The drawing under review shows one solid part. Ordinate dimensions are in mm from its lowest x, y, z. Coordinates: 2 decimals unless noted, no trailing zeros. Write each loop counter-clockwise with the first axis right and the second up, starting at its lowest first coordinate (ties: lowest second). Pieces come first, ordered by that corner, then holes.
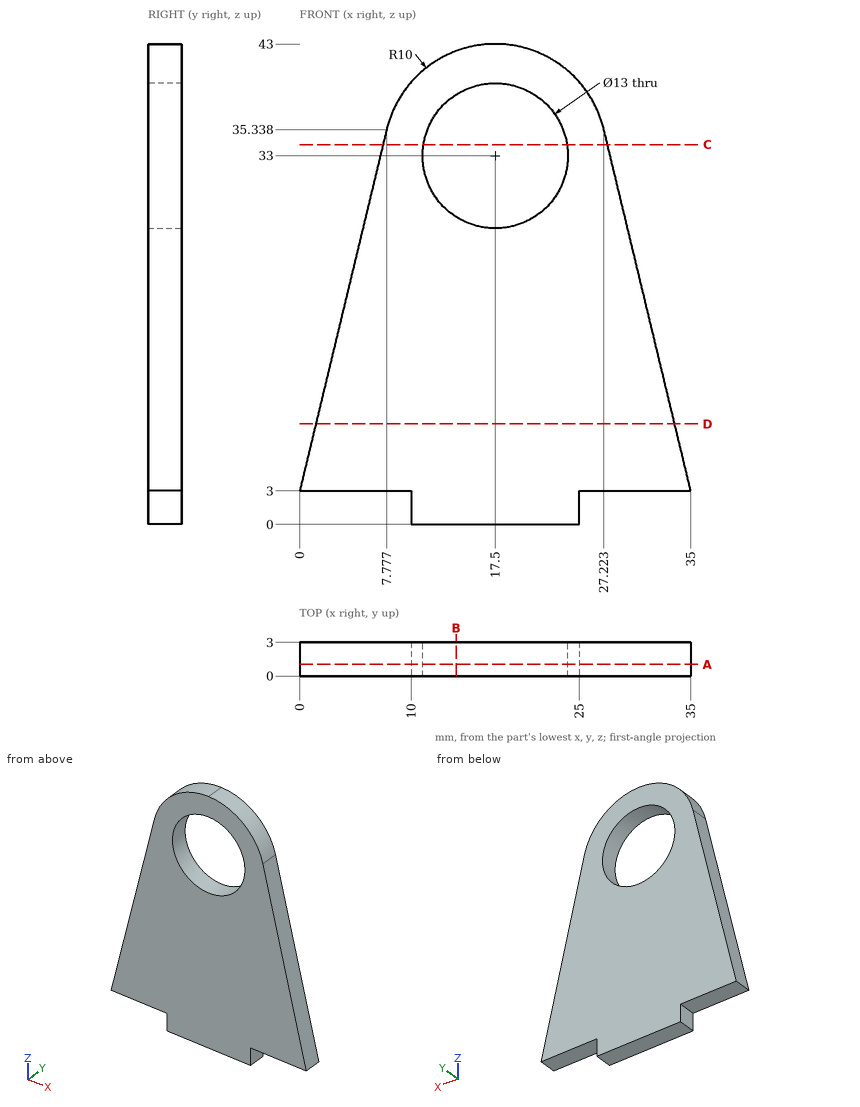
Q1. Add section A-A (y = 1.05). State the section outline as (x, z) points, then the cut area to 3 significant figures.
Ans:
outline: (0, 3) - (10, 3) - (10, 0) - (25, 0) - (25, 3) - (35, 3) - (27.22, 35.34) arc R10 ccw to (17.5, 43) arc R10 ccw to (7.78, 35.34) - close; hole circle Ø13 at (17.5, 33)
area: 903 mm2
Q2. Add section C-C (z = 34). State the section outline as (x, y) points (1 decimal), then the cut area to 3 significant figures.
Ans:
outline: (7.5, 0) - (11.1, 0) - (11.1, 3) - (7.5, 3) - close; (23.9, 0) - (27.5, 0) - (27.5, 3) - (23.9, 3) - close
area: 21.7 mm2
Q3. Add section B-B (x = 14). State the section outline as (y, z) points.
Ans:
outline: (0, 0) - (3, 0) - (3, 27.52) - (0, 27.52) - close; (0, 38.48) - (3, 38.48) - (3, 42.37) - (0, 42.37) - close
Q4. Add section D-D (z = 9). State the section outline as (x, y) points.
Ans:
outline: (1.44, 0) - (33.56, 0) - (33.56, 3) - (1.44, 3) - close
Q5. Clearance check with flat-ended pins moving along their axes: pin 1 Ø0.9 at (y, z) = (1, 1.5) entering from +X; pin 2 Ø0.9 at (x, y) = (31.5, 2) entering from -Z. State where each tip first meets the part, or that it passes through.
Ans:
pin 1: stops at x = 25
pin 2: stops at z = 3
Q6. For probe 1 along X at (y, z) = (0.7, 33) (1 decimal); probe 2 along X at (y, z) = (0.45, 36); probe 3 along X at (y, z) = (1.2, 2), list the stretches that pass through material, from the lowest coordinate up.
Ans:
probe 1: x = 7.2 to 11, 24 to 27.8
probe 2: x = 7.96 to 11.73, 23.27 to 27.04
probe 3: x = 10 to 25
